Verification items for the finished model (mm, model axes). A direction names the side the tool comes from. Coordinates: 2 decimals unless noted, no trailing zeros. Order: outer loops, then holes, each group sorted by start corner. A loop starts at its lowest first (then second) coordinate and runs counter-clockwise, first axis right, second up. Notation, with made-up numbers: M 82.25,10 L 107.25,10 A15 ccw 107.25,28 Z; hole C 26,46 d8. An arc over 180 degrees is marked long. Write item = value, one per line.
```python
from build123d import *

# Parameters (mm, degrees)
SZKIC1_R                    = 1.4
DODANIE_WYCI_GNI_CIE1_DEPTH = 2
SZKIC1_3_W                  = 4.25
SZKIC1_3_H                  = 14
DODANIE_WYCI_GNI_CIE2_DEPTH = 7
DODANIE_WYCI_GNI_CIE3_DEPTH = 7
SZKIC2_W                    = 10
SZKIC2_H                    = 14
DODANIE_WYCI_GNI_CIE4_DEPTH = 3
DODANIE_WYCI_GNI_CIE5_START = 2
SZKIC1_5_W                  = 1
SZKIC1_5_H                  = 7
DODANIE_WYCI_GNI_CIE5_DEPTH = 3.5
DODANIE_WYCI_GNI_CIE6_REACH = 30.417
WYTNIJ_WYCI_GNI_CIE1_REACH  = 27.125
WYTNIJ_WYCI_GNI_CIE2_DEPTH  = 3
SZKIC6_W                    = 2.25
SZKIC6_H                    = 14
WYTNIJ_WYCI_GNI_CIE3_DEPTH  = 1
SZKIC7_W                    = 4
SZKIC7_H                    = 4
DODANIE_WYCI_GNI_CIE7_DEPTH = 4
WYTNIJ_WYCI_GNI_CIE4_DEPTH  = 4
WYTNIJ_WYCI_GNI_CIE5_DEPTH  = 34.841542518


with BuildPart() as part:
    # Szkic1 → Dodanie-wyciągnięcie1 (new body)
    with BuildSketch(Plane(origin=(0, 0, 0), x_dir=(1, 0, 0), z_dir=(0, 1, 0))):
        with BuildLine():
            Line((-17, 3.5), (0, 3.5))
            ThreePointArc((0, 3.5), (3.5, 0), (0, -3.5))
            Line((0, -3.5), (-17, -3.5))
            ThreePointArc((-17, -3.5), (-20.5, 0), (-17, 3.5))
        make_face()
        with Locations(Location((-17, 0, 0), (0, 0, 270))):
            Circle(SZKIC1_R, mode=Mode.SUBTRACT)
        with Locations(Location((0, 0, 0), (0, 0, 270))):
            Circle(SZKIC1_R, mode=Mode.SUBTRACT)
    extrude(amount=DODANIE_WYCI_GNI_CIE1_DEPTH)

    # Szkic1<3> → Dodanie-wyciągnięcie2 (add)
    with BuildSketch(Plane(origin=(0, 0, 0), x_dir=(1, 0, 0), z_dir=(0, 1, 0))):
        with Locations((-13.625, -10.5)):
            Rectangle(SZKIC1_3_W, SZKIC1_3_H)
        Polygon((-10.5, -3.5), (-11.5, -3.5), (-11.5, -17.5), (-5.5, -17.5), (-5.5, -3.5), (-6.5, -3.5), align=None)
        with Locations((-3.375, -10.5)):
            Rectangle(SZKIC1_3_W, SZKIC1_3_H)
    extrude(amount=DODANIE_WYCI_GNI_CIE2_DEPTH)

    # Szkic1<4> → Dodanie-wyciągnięcie3 (add)
    with BuildSketch(Plane(origin=(0, 0, 0), x_dir=(1, 0, 0), z_dir=(0, 1, 0))):
        Polygon((-10.5, -3.5), (-11.5, -3.5), (-11.5, -17.5), (-5.5, -17.5), (-5.5, -3.5), (-6.5, -3.5), align=None)
    extrude(amount=-DODANIE_WYCI_GNI_CIE3_DEPTH)

    # Szkic2 → Dodanie-wyciągnięcie4 (add)
    with BuildSketch(Plane(origin=(0, 7, 0), x_dir=(1, 0, 0), z_dir=(0, 1, 0))):
        with Locations((-8.5, -10.5)):
            Rectangle(SZKIC2_W, SZKIC2_H)
    extrude(amount=DODANIE_WYCI_GNI_CIE4_DEPTH)

    # Szkic1<5> → Dodanie-wyciągnięcie5 (add)
    with BuildSketch(Plane(origin=(0, 0, 0), x_dir=(1, 0, 0), z_dir=(0, 1, 0)).offset(DODANIE_WYCI_GNI_CIE5_START)):
        with Locations((-6, 0)):
            Rectangle(SZKIC1_5_W, SZKIC1_5_H)
        with Locations((-11, 0)):
            Rectangle(SZKIC1_5_W, SZKIC1_5_H)
    extrude(amount=DODANIE_WYCI_GNI_CIE5_DEPTH)

    # Dodanie-wyciągnięcie6: up to this face of the body (flat: up to its plane)
    dodanie_wyci_gni_cie6_end = Plane(part.part.faces().sort_by_distance((-8.5, 10, 10.5))[0])
    # Szkic3 → Dodanie-wyciągnięcie6 (add, up to the picked face)
    with BuildSketch(Plane(origin=(0, 2, 0), x_dir=(1, 0, 0), z_dir=(0, 1, 0)), mode=Mode.PRIVATE) as dodanie_wyci_gni_cie6_sk1:
        Polygon((-3.5, -3.5), (-5.5, -1.5), (-6.5, -1.5), (-6.5, -3.5), (-5.5, -3.5), align=None)
    dodanie_wyci_gni_cie6_tool1 = split(extrude(dodanie_wyci_gni_cie6_sk1.sketch, amount=DODANIE_WYCI_GNI_CIE6_REACH, mode=Mode.PRIVATE), bisect_by=dodanie_wyci_gni_cie6_end, keep=Keep.BOTH, mode=Mode.PRIVATE)
    # Szkic3 → Dodanie-wyciągnięcie6 (add, up to the picked face)
    with BuildSketch(Plane(origin=(0, 2, 0), x_dir=(1, 0, 0), z_dir=(0, 1, 0)), mode=Mode.PRIVATE) as dodanie_wyci_gni_cie6_sk2:
        Polygon((-11.5, -3.5), (-13.5, -3.5), (-11.5, -1.5), (-10.5, -1.5), (-10.5, -3.5), align=None)
    dodanie_wyci_gni_cie6_tool2 = split(extrude(dodanie_wyci_gni_cie6_sk2.sketch, amount=DODANIE_WYCI_GNI_CIE6_REACH, mode=Mode.PRIVATE), bisect_by=dodanie_wyci_gni_cie6_end, keep=Keep.BOTH, mode=Mode.PRIVATE)
    add(dodanie_wyci_gni_cie6_tool1.solids().sort_by(Axis((-5.416667, 2, 2.666667), (0, 1, 0)))[0])
    add(dodanie_wyci_gni_cie6_tool2.solids().sort_by(Axis((-11.583333, 2, 2.666667), (0, 1, 0)))[0])

    # Wytnij-wyciągnięcie1: up to this face of the body (flat: up to its plane)
    wytnij_wyci_gni_cie1_end = Plane(part.part.faces().sort_by_distance((-5.5, 3.75, -1))[0])
    # Szkic4 → Wytnij-wyciągnięcie1 (cut, up to the picked face)
    with BuildSketch(Plane.ZY.offset(11.5), mode=Mode.PRIVATE) as wytnij_wyci_gni_cie1_sk1:
        Polygon((1.5, 5.5), (-3.5, 3), (-3.5, 5.5), align=None)
    wytnij_wyci_gni_cie1_tool1 = split(extrude(wytnij_wyci_gni_cie1_sk1.sketch, amount=-WYTNIJ_WYCI_GNI_CIE1_REACH, mode=Mode.PRIVATE), bisect_by=wytnij_wyci_gni_cie1_end, keep=Keep.BOTH, mode=Mode.PRIVATE)
    add(wytnij_wyci_gni_cie1_tool1.solids().sort_by(Axis((-11.5, 4.666667, -1.833333), (1, 0, 0)))[0], mode=Mode.SUBTRACT)

    # Szkic5 → Wytnij-wyciągnięcie2 (cut)
    with BuildSketch(Plane(origin=(0, 10, 0), x_dir=(1, 0, 0), z_dir=(0, 1, 0))):
        Polygon((-5.45, -17.5), (-3.5, -17.5), (-3.5, -3.5), (-4.600591716, -2.399408284), align=None)
        Polygon((-13.5, -3.5), (-12.399408284, -2.399408284), (-11.55, -17.5), (-13.5, -17.5), align=None)
    extrude(amount=-WYTNIJ_WYCI_GNI_CIE2_DEPTH, mode=Mode.SUBTRACT)

    # Szkic6 → Wytnij-wyciągnięcie3 (cut)
    with BuildSketch(Plane(origin=(0, 7, 0), x_dir=(1, 0, 0), z_dir=(0, 1, 0))):
        with Locations((-2.375, -10.5)):
            Rectangle(SZKIC6_W, SZKIC6_H)
        with Locations((-14.625, -10.5)):
            Rectangle(SZKIC6_W, SZKIC6_H)
    extrude(amount=-WYTNIJ_WYCI_GNI_CIE3_DEPTH, mode=Mode.SUBTRACT)

    # Szkic7 → Dodanie-wyciągnięcie7 (add)
    with BuildSketch(Plane.XY.offset(17.5)):
        with Locations((-8.5, 6.5)):
            Rectangle(SZKIC7_W, SZKIC7_H)
    extrude(amount=DODANIE_WYCI_GNI_CIE7_DEPTH)

    # Szkic8 → Wytnij-wyciągnięcie4 (cut)
    with BuildSketch(Plane(origin=(0, 8.5, 0), x_dir=(1, 0, 0), z_dir=(0, 1, 0))):
        Polygon((-8.1, -21.5), (-6.5, -19), (-6.5, -21.5), align=None)
        Polygon((-8.9, -21.5), (-10.5, -19), (-10.5, -21.5), align=None)
    extrude(amount=-WYTNIJ_WYCI_GNI_CIE4_DEPTH, mode=Mode.SUBTRACT)

    # Szkic9 → Wytnij-wyciągnięcie5 (cut, through all)
    with BuildSketch(Plane.XY.offset(21.5)):
        with BuildLine():
            Line((-7.6, 7.9), (-9.4, 7.9))
            ThreePointArc((-9.4, 7.9), (-9.753553391, 7.753553391), (-9.9, 7.4))
            Line((-9.9, 7.4), (-9.9, 5.6))
            ThreePointArc((-9.9, 5.6), (-9.753553391, 5.246446609), (-9.4, 5.1))
            Line((-9.4, 5.1), (-7.6, 5.1))
            ThreePointArc((-7.6, 5.1), (-7.246446609, 5.246446609), (-7.1, 5.6))
            Line((-7.1, 5.6), (-7.1, 7.4))
            ThreePointArc((-7.1, 7.4), (-7.246446609, 7.753553391), (-7.6, 7.9))
        make_face()
    extrude(amount=-WYTNIJ_WYCI_GNI_CIE5_DEPTH, mode=Mode.SUBTRACT)


solid = part.part
```
Item 1: Release check for a two-part mould opening along X. For faces 6 (the flat face through (-11, 8, 1.5)), 7 (the flat face through (-7.1, 6, 12)), 8 (the flat face through (-13, 5, 3)) record: pulls with the +X half, pulls with the -X half, needs draft (parallel to the pull), parting line crosses it, or undercut.
Report:
face_6 = needs draft
face_7 = undercut
face_8 = pulls with the -X half
Item 2: Sectioned sample at A-A, the plane z = 0. Enter the section's corners in (x, y).
Report:
outline = M -20.5,0 L -18.4,0 L -18.4,2 L -20.5,2 Z; M -15.6,0 L -1.4,0 L -1.4,2 L -5.5,2 L -5.5,4.75 L -6.5,4.75 L -6.5,2 L -10.5,2 L -10.5,4.75 L -11.5,4.75 L -11.5,2 L -15.6,2 Z; M 1.4,0 L 3.5,0 L 3.5,2 L 1.4,2 Z
Item 3: Tool access check on faces 1 (the flat face through (-13.5, 6.5, 10.6)), 2 (the flat face through (-6, 8, 1.5)), 3 (the flat face through (-11.98, 8.52, 9.84)), 4 (the flat face through (-11.5, -3, 10)), 5 (the flat face through (-6.5, 5, 2)). Record the directions out of +Z, -Z, +X, -X, +Y, -Y that give a thin tool (end or side, any length) a straight path to the whole face; none if there is none.
Report:
face_1 = +Z, -Z, -X, +Y
face_2 = -Z, +X, -X, +Y
face_3 = +Z, -X, +Y
face_4 = +Z, -Z, -X, -Y
face_5 = -Z, +Y
Item 4: Scan lines: L1, parallel to X at y = 1.4, z = 0; L2, parallel to Y at x = -7.75, z = 5.5; L3, parallel to X at y = -2, z = 9. Record each from-to range of solid material in increasing order. Write a range as from..to.
Report:
L1 = -20.5..-18.4, -15.6..-1.4, 1.4..3.5
L2 = -7..5.1, 7.9..10
L3 = -11.5..-5.5
Item 5: Sectioned sample at D-D, the plane z = 7. Enter the section's corners in (x, y).
Report:
outline = M -15.75,0 L -11.5,0 L -11.5,-7 L -5.5,-7 L -5.5,0 L -1.25,0 L -1.25,6 L -3.5,6 L -3.5,7 L -4.86,7 L -4.86,10 L -12.14,10 L -12.14,7 L -13.5,7 L -13.5,6 L -15.75,6 Z; hole M -9.9,5.6 A0.5 ccw -9.4,5.1 L -7.6,5.1 A0.5 ccw -7.1,5.6 L -7.1,7.4 A0.5 ccw -7.6,7.9 L -9.4,7.9 A0.5 ccw -9.9,7.4 Z
Item 6: Sectioned sample at B-B, the plane y = 1.5. Enter the section's corners in (x, z), then the cut area to 3 significant figures.
Report:
outline = M -17,-3.5 L 0,-3.5 A3.5 ccw 0,3.5 L -1.25,3.5 L -1.25,17.5 L -15.75,17.5 L -15.75,3.5 L -17,3.5 A3.5 ccw Z; hole C -17,0 d2.8; hole C 0,0 d2.8
area = 348 mm^2
Item 7: Gauge pin test, flat ends, axial feed: pin 1 (10 mm diameter, centred on x = -9, y = -4.5, fed in from +Z); pin 2 (1.4 mm diameter, centred on y = 6, z = 10, fed in from +X); pin 3 (0.8 mm diameter, centred on y = 6.5, z = 18.5, fed in from -X); pin 4 (8 mm diameter, centred on x = -2, z = 0, fed in from +Y). Record the tip position at first contact, or that the pin passes through.
Report:
pin_1 = 17.5
pin_2 = -1.25
pin_3 = -10.5
pin_4 = 10
Item 8: Sectioned sample at C-C, the plane y = 9. Enter the section's corners in (x, z).
Report:
outline = M -12.4,2.4 L -11.5,1.5 L -10.5,1.5 L -10.5,3.5 L -6.5,3.5 L -6.5,1.5 L -5.5,1.5 L -4.6,2.4 L -5.45,17.5 L -11.55,17.5 Z
